```python
from build123d import *

# Parameters (mm, degrees)
F1_DEPTH     = 4.699
F2_R         = 3.175
F3_R         = 1.524
F4_R         = 6.35
F5_T1_DEPTH  = 11.176
F5_T3_DEPTH  = 136.4146354703
F5_T5_DEPTH  = 6.35
F5_T7_DEPTH  = 146.1327814154
F5_S11_W     = 1.524
F5_S11_H     = 1.524
F5_T12_DEPTH = 1.524
F5_S17_W     = 1.524
F5_S17_H     = 1.524
F5_T18_DEPTH = 1.524
F5_T22_ANGLE = 43.7268911646
F5_T24_ANGLE = 43.7268911646
F5_T26_ANGLE = 90
F5_T28_ANGLE = 90
F5_T30_ANGLE = 43.7268911646
F5_T32_ANGLE = 43.7268911646
F5_T34_ANGLE = 90
F5_T36_ANGLE = 90
F6_R         = 2.5781
F7_DEPTH     = 22.9372001


# Not quite as in the source:
# - a fillet or chamfer that OpenCascade refuses, or shapes differently, is made with other operations: its cross-section is extruded or revolved along the edge and cut away or added


with BuildPart() as f1:
    # F0 (on Front) → F1 (new body, symmetric)
    with BuildSketch(Plane.XZ):
        with BuildLine():
            ThreePointArc((0, 21.0312), (11.8754711368, 17.3575504816), (19.6022185846, 7.62))
            Line((19.6022185846, 7.62), (165.1, 7.62))
            Line((165.1, 7.62), (165.1, 20.32))
            Line((165.1, 20.32), (22.8205819041, 20.32))
            ThreePointArc((22.8205819041, 20.32), (12.5055862406, 27.879951062), (0, 30.5562))
            Line((0, 30.5562), (-12.7, 30.5562))
            Line((-12.7, 30.5562), (-12.7, 21.0312))
            Line((-12.7, 21.0312), (0, 21.0312))
        make_face()
    extrude(amount=F1_DEPTH, both=True)

    # F2
    f2_edges = [f1.edges().sort_by_distance(p)[0] for p in [
        (165.1, 0, 20.32),
        (165.1, 0, 7.62),
    ]]
    fillet(f2_edges, radius=F2_R)

    # F3
    f3_edges = [f1.edges().sort_by_distance(p)[0] for p in [
        (-12.7, 4.699, 25.7937),
        (-12.7, 0, 21.0312),
        (-12.7, -4.699, 25.7937),
        (-12.7, 0, 30.5562),
    ]]
    fillet(f3_edges, radius=F3_R)

    # F4
    f4_edges = [f1.edges().sort_by_distance(p)[0] for p in [
        (22.820582, 0, 20.32),
    ]]
    fillet(f4_edges, radius=F4_R)

    # F5: fillet of radius 1.524 on 2 edges, made by hand

    # F5_s2 → F5_t1 (cut)
    with BuildSketch(Plane.YZ.offset(-11.176)):
        with BuildLine():
            ThreePointArc((-3.175, 30.5562), (-4.2526307345, 30.1098307345), (-4.699, 29.0322))
            Line((-4.699, 29.0322), (-4.699, 30.5562))
            Line((-4.699, 30.5562), (-3.175, 30.5562))
        make_face()
        with BuildLine():
            ThreePointArc((4.699, 29.0322), (4.2526307345, 30.1098307345), (3.175, 30.5562))
            Line((3.175, 30.5562), (4.699, 30.5562))
            Line((4.699, 30.5562), (4.699, 29.0322))
        make_face()
    extrude(amount=F5_T1_DEPTH, mode=Mode.SUBTRACT)

    # F5_s4 → F5_t3 (cut)
    with BuildSketch(Plane.YZ.offset(25.5103645297)):
        with BuildLine():
            ThreePointArc((4.699, 18.796), (4.2526307345, 19.8736307345), (3.175, 20.32))
            Line((3.175, 20.32), (4.699, 20.32))
            Line((4.699, 20.32), (4.699, 18.796))
        make_face()
        with BuildLine():
            ThreePointArc((-3.175, 20.32), (-4.2526307345, 19.8736307345), (-4.699, 18.796))
            Line((-4.699, 18.796), (-4.699, 20.32))
            Line((-4.699, 20.32), (-3.175, 20.32))
        make_face()
    extrude(amount=F5_T3_DEPTH, mode=Mode.SUBTRACT)

    # F5_s6 → F5_t5 (cut)
    with BuildSketch(Plane.XY.offset(10.795)):
        with BuildLine():
            ThreePointArc((163.576, 4.699), (164.6536307345, 4.2526307345), (165.1, 3.175))
            Line((165.1, 3.175), (165.1, 4.699))
            Line((165.1, 4.699), (163.576, 4.699))
        make_face()
        with BuildLine():
            ThreePointArc((165.1, -3.175), (164.6536307345, -4.2526307345), (163.576, -4.699))
            Line((163.576, -4.699), (165.1, -4.699))
            Line((165.1, -4.699), (165.1, -3.175))
        make_face()
    extrude(amount=F5_T5_DEPTH, mode=Mode.SUBTRACT)

    # F5_s8 → F5_t7 (cut)
    with BuildSketch(Plane.YZ.offset(15.7922185846)):
        with BuildLine():
            ThreePointArc((4.699, 9.144), (4.2526307345, 8.0663692655), (3.175, 7.62))
            Line((3.175, 7.62), (4.699, 7.62))
            Line((4.699, 7.62), (4.699, 9.144))
        make_face()
        with BuildLine():
            ThreePointArc((-3.175, 7.62), (-4.2526307345, 8.0663692655), (-4.699, 9.144))
            Line((-4.699, 9.144), (-4.699, 7.62))
            Line((-4.699, 7.62), (-3.175, 7.62))
        make_face()
    extrude(amount=F5_T7_DEPTH, mode=Mode.SUBTRACT)


with BuildPart() as f5_tool10:
    # F5_s11 → F5_t12 (new body)
    with BuildSketch(Plane.XZ.offset(-3.175)):
        with Locations((-11.938, 29.7942)):
            Rectangle(F5_S11_W, F5_S11_H)
    extrude(amount=-F5_T12_DEPTH)

    # F5_s13 → F5_t14 (revolve, cut)
    with BuildSketch(Plane(origin=(-11.176, 3.175, 29.0322), x_dir=(0.7071067812, 0, -0.7071067812), z_dir=(0.7071067812, 0, 0.7071067812))):
        with BuildLine():
            ThreePointArc((0, -1.524), (1.524, 0), (0, 1.524))
            Line((0, 1.524), (0, -1.524))
        make_face()
    revolve(axis=Axis((-11.176, 3.175, 29.0322), (0, 1, 0)), mode=Mode.SUBTRACT)


with BuildPart() as f1_1:
    add(f1.part)

    # F5_t9: cut F5_tool10
    add(f5_tool10.part, mode=Mode.SUBTRACT)


with BuildPart() as f5_tool16:
    # F5_s17 → F5_t18 (new body)
    with BuildSketch(Plane.XY.offset(29.0322)):
        with Locations((-11.938, -3.937)):
            Rectangle(F5_S17_W, F5_S17_H)
    extrude(amount=F5_T18_DEPTH)

    # F5_s19 → F5_t20 (revolve, cut)
    with BuildSketch(Plane(origin=(-11.176, -3.175, 29.0322), x_dir=(0.7071067812, 0.7071067812, 0), z_dir=(0.7071067812, -0.7071067812, 0))):
        with BuildLine():
            ThreePointArc((0, -1.524), (1.524, 0), (0, 1.524))
            Line((0, 1.524), (0, -1.524))
        make_face()
    revolve(axis=Axis((-11.176, -3.175, 29.0322), (0, 0, 1)), mode=Mode.SUBTRACT)


with BuildPart() as f1_2:
    add(f1_1.part)

    # F5_t15: cut F5_tool16
    add(f5_tool16.part, mode=Mode.SUBTRACT)

    # F5_s21 → F5_t22 (revolve, cut)
    with BuildSketch(Plane(origin=(0, 0, 0), x_dir=(0, 1, 0), z_dir=(0.722642808, 0, -0.6912216519))):
        with BuildLine():
            ThreePointArc((4.699, 29.0322), (4.2526307345, 30.1098307345), (3.175, 30.5562))
            Line((3.175, 30.5562), (4.699, 30.5562))
            Line((4.699, 30.5562), (4.699, 29.0322))
        make_face()
    revolve(axis=Axis((0, 4.699, 0), (0, -1, 0)), revolution_arc=F5_T22_ANGLE, mode=Mode.SUBTRACT)

    # F5_s23 → F5_t24 (revolve, cut)
    with BuildSketch(Plane(origin=(0, 0, 0), x_dir=(0, 1, 0), z_dir=(-0.722642808, 0, 0.6912216519))):
        with BuildLine():
            ThreePointArc((4.699, -29.0322), (4.2526307345, -30.1098307345), (3.175, -30.5562))
            Line((3.175, -30.5562), (4.699, -30.5562))
            Line((4.699, -30.5562), (4.699, -29.0322))
        make_face()
    revolve(axis=Axis((25.5103645297, 4.699, 26.67), (0, -1, 0)), revolution_arc=F5_T24_ANGLE, mode=Mode.SUBTRACT)

    # F5_s25 → F5_t26 (revolve, cut)
    with BuildSketch(Plane.YZ.offset(161.925)):
        with BuildLine():
            ThreePointArc((4.699, 18.796), (4.2526307345, 19.8736307345), (3.175, 20.32))
            Line((3.175, 20.32), (4.699, 20.32))
            Line((4.699, 20.32), (4.699, 18.796))
        make_face()
    revolve(axis=Axis((161.925, 4.699, 17.145), (0, 1, 0)), revolution_arc=F5_T26_ANGLE, mode=Mode.SUBTRACT)

    # F5_s27 → F5_t28 (revolve, cut)
    with BuildSketch(Plane.XY.offset(10.795)):
        with BuildLine():
            ThreePointArc((163.576, 4.699), (164.6536307345, 4.2526307345), (165.1, 3.175))
            Line((165.1, 3.175), (165.1, 4.699))
            Line((165.1, 4.699), (163.576, 4.699))
        make_face()
    revolve(axis=Axis((161.925, 4.699, 10.795), (0, 1, 0)), revolution_arc=F5_T28_ANGLE, mode=Mode.SUBTRACT)

    # F5_s29 → F5_t30 (revolve, cut)
    with BuildSketch(Plane(origin=(0, 0, 0), x_dir=(0, 1, 0), z_dir=(0.722642808, 0, -0.6912216519))):
        with BuildLine():
            ThreePointArc((-3.175, 30.5562), (-4.2526307345, 30.1098307345), (-4.699, 29.0322))
            Line((-4.699, 29.0322), (-4.699, 30.5562))
            Line((-4.699, 30.5562), (-3.175, 30.5562))
        make_face()
    revolve(axis=Axis((0, -4.699, 0), (0, -1, 0)), revolution_arc=F5_T30_ANGLE, mode=Mode.SUBTRACT)

    # F5_s31 → F5_t32 (revolve, cut)
    with BuildSketch(Plane(origin=(0, 0, 0), x_dir=(0, 1, 0), z_dir=(-0.722642808, 0, 0.6912216519))):
        with BuildLine():
            ThreePointArc((-3.175, -30.5562), (-4.2526307345, -30.1098307345), (-4.699, -29.0322))
            Line((-4.699, -29.0322), (-4.699, -30.5562))
            Line((-4.699, -30.5562), (-3.175, -30.5562))
        make_face()
    revolve(axis=Axis((25.5103645297, -4.699, 26.67), (0, -1, 0)), revolution_arc=F5_T32_ANGLE, mode=Mode.SUBTRACT)

    # F5_s33 → F5_t34 (revolve, cut)
    with BuildSketch(Plane.YZ.offset(161.925)):
        with BuildLine():
            ThreePointArc((-3.175, 20.32), (-4.2526307345, 19.8736307345), (-4.699, 18.796))
            Line((-4.699, 18.796), (-4.699, 20.32))
            Line((-4.699, 20.32), (-3.175, 20.32))
        make_face()
    revolve(axis=Axis((161.925, -4.699, 17.145), (0, 1, 0)), revolution_arc=F5_T34_ANGLE, mode=Mode.SUBTRACT)

    # F5_s35 → F5_t36 (revolve, cut)
    with BuildSketch(Plane.XY.offset(10.795)):
        with BuildLine():
            ThreePointArc((165.1, -3.175), (164.6536307345, -4.2526307345), (163.576, -4.699))
            Line((163.576, -4.699), (165.1, -4.699))
            Line((165.1, -4.699), (165.1, -3.175))
        make_face()
    revolve(axis=Axis((161.925, -4.699, 10.795), (0, 1, 0)), revolution_arc=F5_T36_ANGLE, mode=Mode.SUBTRACT)

    # F6 (on face) → F7 (cut, through all)
    with BuildSketch(Plane.XY.offset(30.5562)):
        Circle(F6_R)
    extrude(amount=-F7_DEPTH, mode=Mode.SUBTRACT)


solid = f1_2.part
```
Here's how the part is built. I have some questions about the finished solid (model axes, mm). A direction names the side the tool comes from. Round coordinates to 2 decimals unless told otherwise and drop trailing zeros. Order: outer loops, then holes, each group sorted by start corner. A loop starts at its lowest first (then second) coordinate and runs counter-clockwise, first axis right, second up. Notation, with made-up numbers: M 25.25,51.25 L 40.25,51.25 A24 cw 40.25,73.25 Z; hole C 45.5,20 d2. An arc over 180 degrees is marked long. Answer in a Markdown table with one row per item.
Item 1: If I drill on L1, parallel to Y at x = 0, z = 25.75; L2, parallel to Z at x = 62.5, y = 3; L3, parallel to X at y = 0, z = 27.25, over which ranges is the centre line in solid material (lowest first)? Write a range as from..to.
A:
| item | result |
|---|---|
| L1 | y = -4.7..-2.58, 2.58..4.7 |
| L2 | z = 7.62..20.32 |
| L3 | x = -12.7..-2.58, 2.58..13.82 |
Item 2: Imagine slicing it at A-A, the plane y = 0. Write out the boundary of the cut face in (x, z) (3 decimals), and give its area (3 significant figures).
A:
| item | result |
|---|---|
| outline | M -12.7,22.555 A1.524 ccw -11.176,21.031 L -2.578,21.031 L -2.578,30.556 L -11.176,30.556 A1.524 ccw -12.7,29.032 Z; M 2.578,20.873 A21.031 cw 19.602,7.62 L 161.925,7.62 A3.175 ccw 165.1,10.795 L 165.1,17.145 A3.175 ccw 161.925,20.32 L 25.51,20.32 A6.35 cw 21.121,22.081 A30.556 ccw 2.578,30.447 Z |
| area | 2,140 mm2 |
Item 3: Imagine slicing it at B-B, the plane x = 151. Write out the boundary of the cut face in (y, z) (3 decimals), and give its area (3 significant figures).
A:
| item | result |
|---|---|
| outline | M -4.699,9.144 A1.524 ccw -3.175,7.62 L 3.175,7.62 A1.524 ccw 4.699,9.144 L 4.699,18.796 A1.524 ccw 3.175,20.32 L -3.175,20.32 A1.524 ccw -4.699,18.796 Z |
| area | 117 mm2 |
Item 4: Thinking about a two-plate mould opening in X: for faces 1 (the face through (95, 0, 20.32)), 2 (the face through (164.19, -0.04, 8.57)), 3 (the face through (1.39, 2.17, 25.78)), which applies, +X half, -X half, draft (parallel to the pull), parting line (faces both ways), or undercut?
A:
| item | result |
|---|---|
| face 1 | draft |
| face 2 | +X half |
| face 3 | undercut |
Item 5: I'm going to push flat-ended pins straight in: pin 1 (5 mm diameter, centred on x = 67, y = 1.5, fed in from +Z); pin 2 (2 mm diameter, centred on x = 106.5, z = 20, fed in from -Y). Where does each tip first touch, or does it pass through?
A:
| item | result |
|---|---|
| pin 1 | stops at z = 20.32 |
| pin 2 | stops at y = -4.69 |
Item 6: Imagine slicing it at C-C, the plane z = 15. Write out the boundary of the cut face in (x, y) (3 decimals), and give its area (3 significant figures).
A:
| item | result |
|---|---|
| outline | M 14.741,-4.699 L 163.576,-4.699 A1.524 ccw 165.1,-3.175 L 165.1,3.175 A1.524 ccw 163.576,4.699 L 14.741,4.699 Z |
| area | 1,410 mm2 |
Item 7: For faces 4 (the face through (-6, 0, 21.031)), 5 (the face through (-12.7, 0, 26)), which set-ups out of +Z, -Z, +X, -X, +Y, -Y let a thin tool reach every point of the face, with its end or its side?
A:
| item | result |
|---|---|
| face 4 | -Z, -X, +Y, -Y |
| face 5 | +Z, -Z, -X, +Y, -Y |
